CAD build for the part. Positions are in the model's coordinates, mm. A direction names the side the tool comes from. Round coordinates to 2 decimals unless told otherwise and drop trailing zeros. Order: outer loops, then holes, each group sorted by start corner. A loop starts at its lowest first (then second) coordinate and runs counter-clockwise, first axis right, second up. Notation, with made-up numbers: M 2.25,9.5 L 33.25,9.5 A8 ccw 33.25,13.5 Z; hole C 31.25,37.25 d11. An arc over 180 degrees is marked long. Put each result on its own line as item: value.
```python
from build123d import *

# Parameters (mm, degrees)
SKETCH1_W           = 46.482
SKETCH1_H           = 40.132
BOSS_EXTRUDE1_DEPTH = 1.27
SKETCH2_W           = 11.6205
SKETCH2_H           = 6.35
SKETCH2_W_2         = 6.35
SKETCH2_H_2         = 13.377333334
BOSS_EXTRUDE2_DEPTH = 2.54
SKETCH3_R           = 1.5
SKETCH3_R_2         = 4.953
CUT_EXTRUDE1_DEPTH  = 3.54


with BuildPart() as part:
    # Sketch1 → Boss-Extrude1 (new body, symmetric)
    with BuildSketch(Plane.XY):
        Rectangle(SKETCH1_W, SKETCH1_H)
    extrude(amount=BOSS_EXTRUDE1_DEPTH, both=True)

    # Sketch2 → Boss-Extrude2 (add, through all)
    with BuildSketch(Plane.XY.offset(1.27)):
        with Locations((-17.43075, 23.241)):
            Rectangle(SKETCH2_W, SKETCH2_H)
        with Locations((17.43075, 23.241)):
            Rectangle(SKETCH2_W, SKETCH2_H)
        with Locations((-26.416, 0)):
            Rectangle(SKETCH2_W_2, SKETCH2_H_2)
        with Locations((26.416, 0)):
            Rectangle(SKETCH2_W_2, SKETCH2_H_2)
        with Locations((-17.43075, -23.241)):
            Rectangle(SKETCH2_W, SKETCH2_H)
        with Locations((17.43075, -23.241)):
            Rectangle(SKETCH2_W, SKETCH2_H)
    extrude(amount=-BOSS_EXTRUDE2_DEPTH)

    # Sketch3 → Cut-Extrude1 (cut, through all)
    with BuildSketch(Plane.XY.offset(1.27)):
        with Locations((0, 9.954)):
            Circle(SKETCH3_R)
        with Locations((0, -10.16)):
            Circle(SKETCH3_R_2)
        with Locations((-11.75, -10.397596989)):
            Circle(SKETCH3_R)
        with Locations((11.75, -10.397596989)):
            Circle(SKETCH3_R)
    extrude(amount=-CUT_EXTRUDE1_DEPTH, mode=Mode.SUBTRACT)


solid = part.part
```
Item 1: Band-saw the part on D-D on y = 15.5. Give the cut face in (x, z).
Answers below:
outline: M -23.24,-1.27 L 23.24,-1.27 L 23.24,1.27 L -23.24,1.27 Z
Item 2: Band-saw the part on A-A on x = 0. Give the cut face in (y, z).
Answers below:
outline: M -20.07,-1.27 L -15.11,-1.27 L -15.11,1.27 L -20.07,1.27 Z; M -5.21,-1.27 L 8.45,-1.27 L 8.45,1.27 L -5.21,1.27 Z; M 11.45,-1.27 L 20.07,-1.27 L 20.07,1.27 L 11.45,1.27 Z
Item 3: Mould opens along X. For faces 6 (the flat face through (23.241, 16, 0)), 7 (the flat face through (11.62, -23, 0)), 8 (the flat face through (17, 26.416, 0)), 9 (the cylindrical face through (10.644, -9.384, 0.018)) say: pulls with the +X half, pulls with the -X half, needs draft (parallel to the pull), parting line crosses it, or undercut.
Answers below:
face 6: pulls with the +X half
face 7: undercut
face 8: needs draft
face 9: undercut
Item 4: Tool access for faces 1 (the flat face through (0, -20.066, 0)), 2 (the flat face through (-11.62, 23, 0)), 3 (the flat face through (-23.241, 16, 0)), 4 (the flat face through (26, 6.689, 0)), 5 (the flat face through (26, -6.689, 0)): list every direction of +Z, -Z, +X, -X, +Y, -Y with a clear straight run to the whole face (end or side of a thin tool).
Answers below:
face 1: +Z, -Z, -Y
face 2: +Z, -Z, +Y
face 3: +Z, -Z, -X, +Y
face 4: +Z, -Z, +X, +Y
face 5: +Z, -Z, +X, -Y
Item 5: Pin check, flat tips, straight feed: P1, Ø0.8, axis at y = 14, z = -0.5, coming from the +X side; P2, Ø0.8, axis at y = -23, z = -0.5, coming from the -X side; P3, Ø1.3, axis at x = 0, z = 0, coming from the +Y side; P4, Ø2.5, axis at x = -11.75, y = -10.4, coming from the -Z side. Stop position of each tip, or through.
Answers below:
P1: x = 23.24
P2: x = -23.24
P3: y = 20.07
P4: through
Item 6: Band-saw the part on B-B on y = -7.5. Give the cut face in (x, z), and give its area (3 significant figures).
Answers below:
outline: M -23.24,-1.27 L -4.18,-1.27 L -4.18,1.27 L -23.24,1.27 Z; M 4.18,-1.27 L 23.24,-1.27 L 23.24,1.27 L 4.18,1.27 Z
area: 96.8 mm²
Item 7: Band-saw the part on C-C on z = 0.2. Give the cut face in (x, y), and give its area (3 significant figures).
Answers below:
outline: M -29.59,-6.69 L -23.24,-6.69 L -23.24,-26.42 L -11.62,-26.42 L -11.62,-20.07 L 11.62,-20.07 L 11.62,-26.42 L 23.24,-26.42 L 23.24,-6.69 L 29.59,-6.69 L 29.59,6.69 L 23.24,6.69 L 23.24,26.42 L 11.62,26.42 L 11.62,20.07 L -11.62,20.07 L -11.62,26.42 L -23.24,26.42 L -23.24,6.69 L -29.59,6.69 Z; hole C -11.75,-10.4 d3; hole C 0,-10.16 d9.91; hole C 0,9.95 d3; hole C 11.75,-10.4 d3
area: 2,230 mm²
Item 8: Probe line 1 along Y through (x, z) = (0, 1.1); line 2 along X through (y, z) = (21, -0.8); line 3 along Y through (x, z) = (11.75, -0.35). List the from-to ranges inside material, lowest first. Write a range as [from, to].
Answers below:
line 1: [-20.07, -15.11], [-5.21, 8.45], [11.45, 20.07]
line 2: [-23.24, -11.62], [11.62, 23.24]
line 3: [-26.42, -11.9], [-8.9, 26.42]
